The model under review builds one solid part; all positions refer to its coordinate system, in mm. Face numbers are marked on the shaded views. Coordinates: 2 decimals unless noted, no trailing zeros. Write each loop counter-clockwise with the first axis right and the second up, starting at its lowest first coordinate (ties: lowest second). Pieces come first, ordered by that corner, then holes.
```python
from build123d import *

# Parameters (mm, degrees)
F1_DEPTH = 19.05
F2_DEPTH = 3.175
F3_R     = 4.04114
F4_DEPTH = 25.4


with BuildPart() as f1:
    # F0 (on Top) → F1 (new body)
    with BuildSketch(Plane.XY):
        with BuildLine():
            Line((20.623783, -38.1), (50.8, -38.1))
            Line((50.8, -38.1), (50.8, 38.1))
            Line((50.8, 38.1), (22.225, 38.1))
            Line((22.225, 38.1), (22.225, 21.209))
            ThreePointArc((22.225, 21.209), (22.596974, 20.310974), (23.495, 19.939))
            Line((23.495, 19.939), (31.75, 19.939))
            ThreePointArc((31.75, 19.939), (37.170064, 22.184064), (34.925, 16.764))
            Line((34.925, 16.764), (34.925, -28.448))
            ThreePointArc((34.925, -28.448), (37.170064, -33.868064), (31.75, -31.623))
            Line((31.75, -31.623), (-31.75, -31.623))
            ThreePointArc((-31.75, -31.623), (-37.170064, -33.868064), (-34.925, -28.448))
            Line((-34.925, -28.448), (-34.925, 16.764))
            ThreePointArc((-34.925, 16.764), (-37.170064, 22.184064), (-31.75, 19.939))
            Line((-31.75, 19.939), (-23.495, 19.939))
            ThreePointArc((-23.495, 19.939), (-22.596974, 20.310974), (-22.225, 21.209))
            Line((-22.225, 21.209), (-22.225, 38.1))
            Line((-22.225, 38.1), (-50.8, 38.1))
            Line((-50.8, 38.1), (-50.8, -38.1))
            Line((-50.8, -38.1), (-20.623783, -38.1))
            Line((-20.623783, -38.1), (20.623783, -38.1))
        make_face()
        with BuildLine():
            Line((22.225, 21.209), (22.225, 38.1))
            Line((22.225, 38.1), (-22.225, 38.1))
            Line((-22.225, 38.1), (-22.225, 21.209))
            ThreePointArc((-22.225, 21.209), (-22.596974, 20.310974), (-23.495, 19.939))
            Line((-23.495, 19.939), (-31.75, 19.939))
            ThreePointArc((-31.75, 19.939), (-37.170064, 22.184064), (-34.925, 16.764))
            Line((-34.925, 16.764), (-34.925, -28.448))
            ThreePointArc((-34.925, -28.448), (-37.170064, -33.868064), (-31.75, -31.623))
            Line((-31.75, -31.623), (31.75, -31.623))
            ThreePointArc((31.75, -31.623), (37.170064, -33.868064), (34.925, -28.448))
            Line((34.925, -28.448), (34.925, 16.764))
            ThreePointArc((34.925, 16.764), (37.170064, 22.184064), (31.75, 19.939))
            Line((31.75, 19.939), (23.495, 19.939))
            ThreePointArc((23.495, 19.939), (22.596974, 20.310974), (22.225, 21.209))
        make_face()
    extrude(amount=-F1_DEPTH)

    # F0 (on Top) → F2 (cut)
    with BuildSketch(Plane.XY):
        with BuildLine():
            Line((22.225, 21.209), (22.225, 38.1))
            Line((22.225, 38.1), (-22.225, 38.1))
            Line((-22.225, 38.1), (-22.225, 21.209))
            ThreePointArc((-22.225, 21.209), (-22.596974, 20.310974), (-23.495, 19.939))
            Line((-23.495, 19.939), (-31.75, 19.939))
            ThreePointArc((-31.75, 19.939), (-37.170064, 22.184064), (-34.925, 16.764))
            Line((-34.925, 16.764), (-34.925, -28.448))
            ThreePointArc((-34.925, -28.448), (-37.170064, -33.868064), (-31.75, -31.623))
            Line((-31.75, -31.623), (31.75, -31.623))
            ThreePointArc((31.75, -31.623), (37.170064, -33.868064), (34.925, -28.448))
            Line((34.925, -28.448), (34.925, 16.764))
            ThreePointArc((34.925, 16.764), (37.170064, 22.184064), (31.75, 19.939))
            Line((31.75, 19.939), (23.495, 19.939))
            ThreePointArc((23.495, 19.939), (22.596974, 20.310974), (22.225, 21.209))
        make_face()
    extrude(amount=-F2_DEPTH, mode=Mode.SUBTRACT)

    # F3 (on face) → F4 (cut)
    with BuildSketch(Plane.XY.offset(-3.175)):
        with BuildLine():
            ThreePointArc((14.50594, 30.099), (10.4648, 34.14014), (6.42366, 30.099))
            ThreePointArc((6.42366, 30.099), (10.4648, 26.05786), (14.50594, 30.099))
        make_face()
        with Locations((-10.4648, 30.099)):
            Circle(F3_R)
    extrude(amount=-F4_DEPTH, mode=Mode.SUBTRACT)


solid = f1.part
```
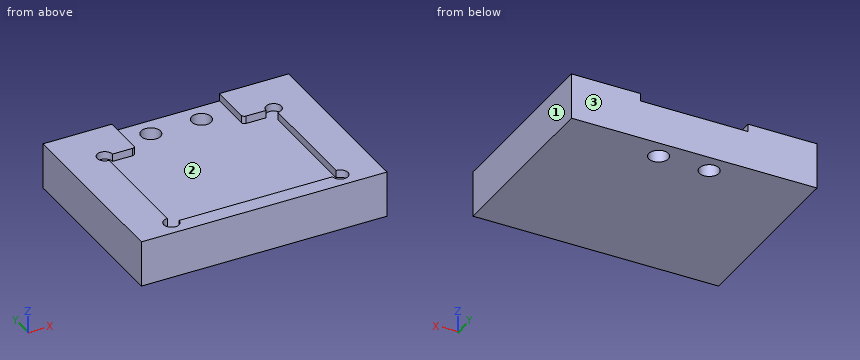
Item 1: To check wall thickness, follow line 1 along X through (y, z) = (-6, -3) (3 decimals); line 2 along Y through (x, z) = (10.5, -16.5); line 3 along Y through (x, z) = (-28.5, -2.75). State the ranges of each line that lie inside material, in increasing order.
Solved:
line 1: x = -50.8 to -34.925, 34.925 to 50.8
line 2: y = -38.1 to 26.06, 34.14 to 38.1
line 3: y = -38.1 to -31.62, 19.94 to 38.1
Item 2: Take a section at B-B, the plane y = -15.5. Write out the cut boundary in (x, z) (3 decimals), plus the area to 3 significant figures.
Solved:
outline: (-50.8, -19.05) - (50.8, -19.05) - (50.8, 0) - (34.925, 0) - (34.925, -3.175) - (-34.925, -3.175) - (-34.925, 0) - (-50.8, 0) - close
area: 1,710 mm2
Item 3: Mouldability with a two-part tool opening along Y and no side actions: class the marked faces 1, 2 and 3 as pulls with the +Y half, pulls with the -Y half, needs draft (parallel to the pull), parting line crosses it, or undercut.
Solved:
face 1: needs draft
face 2: undercut
face 3: pulls with the +Y half
Item 4: Take a section at A-A, the plane x = 25.5. Write out the cut boundary in (y, z) (3 decimals).
Solved:
outline: (-38.1, -19.05) - (38.1, -19.05) - (38.1, 0) - (19.939, 0) - (19.939, -3.175) - (-31.623, -3.175) - (-31.623, 0) - (-38.1, 0) - close
Item 5: Take a section at C-C, the plane x = 12. Write out the cut boundary in (y, z) (3 decimals), plus the area to 3 significant figures.
Solved:
outline: (-38.1, -19.05) - (26.361, -19.05) - (26.361, -3.175) - (-31.623, -3.175) - (-31.623, 0) - (-38.1, 0) - close; (33.837, -19.05) - (38.1, -19.05) - (38.1, -3.175) - (33.837, -3.175) - close
area: 1,110 mm2
Item 6: For pin 1 (1 mm diameter, centred on x = 15.5, z = -1.5, fed in from +Y); pin 2 (10 mm diameter, centred on x = -27, y = -20, fed in from +Z) (3 decimals), all flat-tipped, find the tip position at first contact; note any pin that passes through.
Solved:
pin 1: stops at y = -31.62
pin 2: stops at z = -3.175
Item 7: Take a section at D-D, the plane x = -8. Write out the cut boundary in (y, z) (3 decimals).
Solved:
outline: (-38.1, -19.05) - (26.897, -19.05) - (26.897, -3.175) - (-31.623, -3.175) - (-31.623, 0) - (-38.1, 0) - close; (33.301, -19.05) - (38.1, -19.05) - (38.1, -3.175) - (33.301, -3.175) - close
